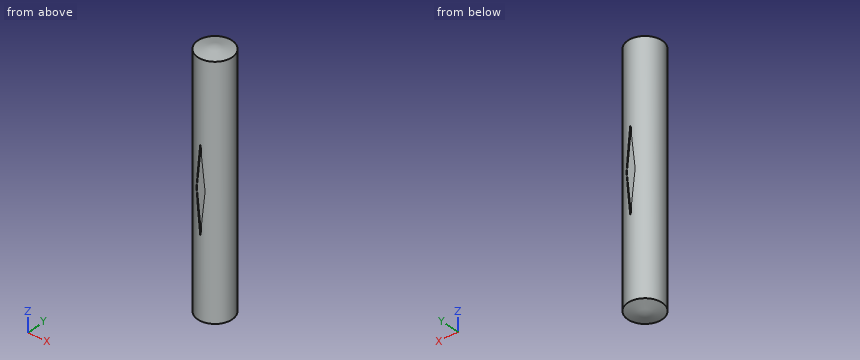
from build123d import *

# Parameters (mm, degrees)
F0_R       = 2
F1_DEPTH   = 29
F2_SIZE2   = 0.3526539614
F2_SIZE    = 2
F2_2_SIZE2 = 0.3526539614
F2_2_SIZE  = 2
F5_DEPTH   = 0.1


# Not quite as in the source:
# - a pattern or mirror of a feature is missing from the dataset's text; its kind, count and spacing are read off the source's solid


with BuildPart() as f1:
    # F0 (on Top) → F1 (new body)
    with BuildSketch(Plane.XY):
        Circle(F0_R)
    extrude(amount=F1_DEPTH)

    # F2
    f2_edges = [f1.edges().sort_by_distance(p)[0] for p in [
        (-2, 0, 29),
    ]]
    f2_side = f1.faces().sort_by_distance((0, 0, 29))[0]
    chamfer(f2_edges, length=F2_SIZE, length2=F2_SIZE2, reference=f2_side)

    # F2#2
    f2_2_edges = [f1.edges().sort_by_distance(p)[0] for p in [
        (-2, 0, 0),
    ]]
    f2_2_side = f1.faces().sort_by_distance((0, 0, 0))[0]
    chamfer(f2_2_edges, length=F2_2_SIZE, length2=F2_2_SIZE2, reference=f2_2_side)

    # F4 (on offset) → F5 (cut)
    with BuildSketch(Plane.XZ.offset(2)):
        Polygon((0.5, 14.5), (0, 19.5), (-0.5, 14.5), (0, 9.5), align=None)
    f5 = extrude(amount=-F5_DEPTH, mode=Mode.SUBTRACT)

    # F5_copies: F5 across plane
    add(f5.mirror(Plane.ZX), mode=Mode.SUBTRACT)


solid = f1.part
Here's how the part is built. I have some questions about the finished solid (model axes, mm). Give positions to 0.01 mm unless a question says otherwise; leave off trailing zeros. Order: outer loops, then holes, each group sorted by start corner. A loop starts at its lowest first (then second) coordinate and runs counter-clockwise, first axis right, second up. Notation, with made-up numbers: M 85.5,11.25 L 144.5,11.25 A22 cw 144.5,28.25 Z; hole C 71.25,-36 d4. An arc over 180 degrees is marked long. Answer as a JSON object with one key per item and string values. Group by question number.
1) I'm going to push flat-ended pins straight in: pin 1 Ø1.5 at (x, y) = (-1.5, -1.5) entering from -Z; pin 2 Ø1 at (y, z) = (-1, 18) entering from -X; pin 3 Ø0.8 at (x, z) = (0, 14) entering from -Y. Where does each tip first touch, or does it pass through?
2) Suppose I cut it at A-A, the plane z = 15.25. Write out the boundary of the cut face in (x, y) (3 decimals), plus the area to 3 significant figures.
3) Please list where these lines run through material, in increasing order: L1, parallel to X at y = 0.15, z = 12; L2, parallel to Z at x = 0.8, y = -1.3; L3, parallel to X at y = -1.4, z = 4.25. Write a range as [from, to].
Results found:
{
 "1": {"pin 1": "z = 0.24", "pin 2": "x = -1.94", "pin 3": "y = -1.9"},
 "2": {"outline": "M -0.425,-1.954 L -0.425,-1.9 L 0.425,-1.9 L 0.425,-1.954 A2 ccw 0.425,1.954 L 0.425,1.9 L -0.425,1.9 L -0.425,1.954 A2 ccw Z", "area": "12.4 mm²"},
 "3": {"L1": "[-1.99, 1.99]", "L2": "[0.27, 28.73]", "L3": "[-1.43, 1.43]"}
}
